Input: part model. Units: mm. Frame: model coordinates. A direction names the side the tool comes from. Coordinates: 2 decimals unless noted, no trailing zeros. Write each loop counter-clockwise with the first axis right and the second up, starting at its lowest first coordinate (ties: lowest second). Pieces come first, ordered by that corner, then holes.
1) Section query C-C (z = 11). Output: boundary loops of the cut face in (x, y), then the cut area to 3 significant figures.
2) Line query: L1, parallel to Z at x = -14.5, y = 3. Output: solid intervals per line, ascending.
3) Set-up query: faces 4 (the flat face through (-25, 6, 10)), 5 (the flat face through (-25, 30, 11)). Return all of +Z, -Z, +X, -X, +Y, -Y with unobstructed straight access to the full face (end or side cutting, diameter ignored); none if empty.
4) Section query A-A (y = 8.75). Output: boundary loops of the cut face in (x, z).
5) Section query B-B (x = -23). Output: boundary loops of the cut face in (y, z), then the cut area to 3 significant figures.
6) Draft query along Z for faces 1 (the flat face through (-25, 15, 0)), 2 (the flat face through (-25, 6, 12)), 3 (the flat face through (-25, 15, 22)). Return one class per face: pulls with the +Z half, pulls with the -Z half, needs draft (parallel to the pull), parting line crosses it, or undercut.
from build123d import *

# Parameters (mm, degrees)
F0_W     = 30
F0_H     = 30
F0_W_2   = 50
F1_DEPTH = 12
F2_W     = 12
F2_H     = 30
F2_H_2   = 12
F2_W_2   = 50
F3_DEPTH = 3.5
F4_W     = 50
F4_H     = 12
F4_W_2   = 12
F4_H_2   = 30
F4_H_3   = 18
F4_W_3   = 18
F5_DEPTH = 10
F6_DEPTH = 10
F7_W     = 30
F7_H     = 65.1035520434
F8_DEPTH = 25


with BuildPart() as f1:
    # F0 (on Top) → F1 (new body)
    with BuildSketch(Plane.XY):
        with Locations((15, -15)):
            Rectangle(F0_W, F0_H)
        with BuildLine():
            Line((0, 30), (0, 0))
            Line((0, 0), (30, 0))
            Line((30, 0), (16.1747587326, 13.8252412674))
            ThreePointArc((16.1747587326, 13.8252412674), (12.3110554274, 14.8605174478), (11.275779247, 18.724220753))
            Line((11.275779247, 18.724220753), (0, 30))
        make_face()
        with Locations((-25, 15)):
            Rectangle(F0_W_2, F0_H)
    extrude(amount=F1_DEPTH)

    # F2 (on face) → F3 (cut)
    with BuildSketch(Plane.XY.offset(12)):
        with Locations((6, -15)):
            Rectangle(F2_W, F2_H)
        with Locations((6, 6)):
            Rectangle(F2_W, F2_H_2)
        with Locations((-25, 6)):
            Rectangle(F2_W_2, F2_H_2)
    extrude(amount=-F3_DEPTH, mode=Mode.SUBTRACT)

    # F4 (on face) → F5 (join)
    with BuildSketch(Plane.XY.offset(12)):
        with Locations((-25, 6)):
            Rectangle(F4_W, F4_H)
        with Locations((6, -15)):
            Rectangle(F4_W_2, F4_H_2)
        with BuildLine():
            Line((11.275779247, 18.724220753), (0, 30))
            Line((0, 30), (0, 12))
            Line((0, 12), (12, 12))
            Line((12, 12), (12, 0))
            Line((12, 0), (30, 0))
            Line((30, 0), (16.1747587326, 13.8252412674))
            ThreePointArc((16.1747587326, 13.8252412674), (12.3110554274, 14.8605174478), (11.275779247, 18.724220753))
        make_face()
        with Locations((6, 6)):
            Rectangle(F4_W_2, F4_H)
        with Locations((-25, 21)):
            Rectangle(F4_W, F4_H_3)
        with Locations((21, -15)):
            Rectangle(F4_W_3, F4_H_2)
    extrude(amount=F5_DEPTH)

    # F0 (on Top) → F6 (join)
    with BuildSketch(Plane.XY):
        with Locations((-25, 15)):
            Rectangle(F0_W_2, F0_H)
        with BuildLine():
            Line((0, 30), (0, 0))
            Line((0, 0), (30, 0))
            Line((30, 0), (16.1747587326, 13.8252412674))
            ThreePointArc((16.1747587326, 13.8252412674), (12.3110554274, 14.8605174478), (11.275779247, 18.724220753))
            Line((11.275779247, 18.724220753), (0, 30))
        make_face()
        with Locations((15, -15)):
            Rectangle(F0_W, F0_H)
        with BuildLine():
            ThreePointArc((19.1394825522, 17.6889445726), (15.6615873211, 21.6547240181), (11.275779247, 18.724220753))
            Line((11.275779247, 18.724220753), (13.7252689898, 16.2747310102))
            Line((13.7252689898, 16.2747310102), (16.1747587326, 13.8252412674))
            ThreePointArc((16.1747587326, 13.8252412674), (18.3128959133, 15.2538988565), (19.1394825522, 17.6889445726))
        make_face()
        with BuildLine():
            ThreePointArc((17.1394825522, 17.6889445726), (15.9048494169, 15.8411855075), (13.7252689898, 16.2747310102))
            ThreePointArc((13.7252689898, 16.2747310102), (14.3741156874, 19.5367036376), (17.1394825522, 17.6889445726))
        make_face(mode=Mode.SUBTRACT)
        with BuildLine():
            Line((13.7252689898, 16.2747310102), (11.275779247, 18.724220753))
            ThreePointArc((11.275779247, 18.724220753), (12.3110554274, 14.8605174478), (16.1747587326, 13.8252412674))
            Line((16.1747587326, 13.8252412674), (13.7252689898, 16.2747310102))
        make_face()
    extrude(amount=F6_DEPTH)

    # F7 (on face) → F8 (cut)
    with BuildSketch(Plane.XY.offset(22)):
        with Locations((15, -2.5517760217)):
            Rectangle(F7_W, F7_H)
    extrude(amount=-F8_DEPTH, mode=Mode.SUBTRACT)


solid = f1.part
Answer:
1. outline: (-50, 12) - (0, 12) - (0, 30) - (-50, 30) - close
1. area: 900 mm2
2. L1: z = 0 to 10, 12 to 22
3. face 4: +X, -X, -Y
3. face 5: +Z, -Z, +X, -X, +Y
4. outline: (-50, 0) - (0, 0) - (0, 10) - (-50, 10) - close; (-50, 12) - (0, 12) - (0, 22) - (-50, 22) - close
5. outline: (0, 0) - (30, 0) - (30, 22) - (0, 22) - (0, 12) - (12, 12) - (12, 10) - (0, 10) - close
5. area: 636 mm2
6. face 1: pulls with the -Z half
6. face 2: undercut
6. face 3: pulls with the +Z half
